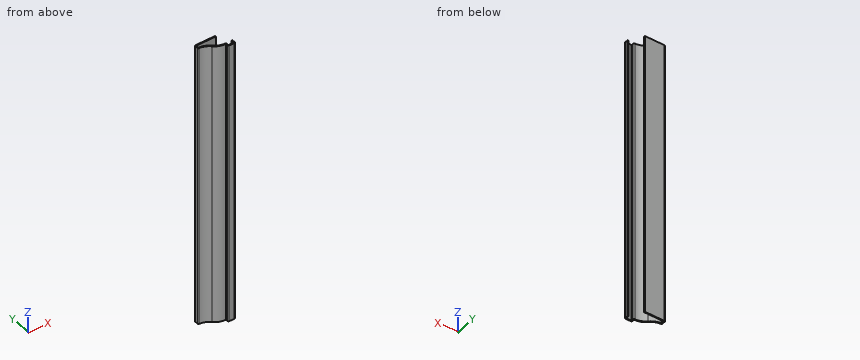
from build123d import *

# Parameters (mm, degrees)
EXTRUDE_THIN1_DEPTH = 285.75
FILLET1_R           = 0.889


with BuildPart() as part:
    # Sketch1 → Extrude-Thin1 (new body)
    with BuildSketch(Plane.XY):
        with BuildLine():
            Line((0, 3.96875), (0, 0))
            Line((0, 0), (-7.14375, 0))
            Line((-7.14375, 0), (-7.14375, 3.175))
            ThreePointArc((-7.14375, 3.175), (-12.992038746, 4.269087389), (-17.962061345, 7.539925789))
            ThreePointArc((-17.962061345, 7.539925789), (-22.83698523, 10.772017174), (-28.575, 11.90625))
            Line((-28.575, 11.90625), (-28.575, 16.66875))
            Line((-28.575, 16.66875), (-7.9375, 16.66875))
            Line((-7.9375, 16.66875), (-7.9375, 15.77975))
            Line((-7.9375, 15.77975), (-27.686, 15.77975))
            Line((-27.686, 15.77975), (-27.686, 12.770487263))
            ThreePointArc((-27.686, 12.770487263), (-22.089870787, 11.419244899), (-17.33645654, 8.171542467))
            ThreePointArc((-17.33645654, 8.171542467), (-12.238465129, 4.931402679), (-6.25475, 4.104858346))
            Line((-6.25475, 4.104858346), (-6.25475, 0.889))
            Line((-6.25475, 0.889), (-0.889, 0.889))
            Line((-0.889, 0.889), (-0.889, 3.96875))
            Line((-0.889, 3.96875), (0, 3.96875))
        make_face()
    extrude(amount=-EXTRUDE_THIN1_DEPTH)

    # Fillet1
    fillet1_edges = [part.edges().sort_by_distance(p)[0] for p in [
        (-6.25475, 4.104858346, -142.875),
        (0, 0, -142.875),
        (-7.14375, 0, -142.875),
        (-28.575, 11.90625, -142.875),
        (-28.575, 16.66875, -142.875),
    ]]
    fillet(fillet1_edges, radius=FILLET1_R)


solid = part.part
Check sheet for the modelled part. Datum: model origin and axes. Units: mm. Give positions to 0.01 mm unless a question says otherwise; leave off trailing zeros. Loops run counter-clockwise (first coordinate to the right, second up) from the corner with the lowest first, then second, coordinate; pieces in that order, holes last. Notation, with made-up numbers: M 89.5,44.25 L 134.5,44.25 A27 cw 134.5,80.25 Z; hole C 85,36.25 d10. An arc over 180 degrees is marked long. Answer as a JSON object with one key per item and string values. Group by question number.
Q1. Material ranges on line 1 along Y through (x, z) = (-8.5, -105.5); line 2 along Y through (x, z) = (-27.25, -38.5); line 3 along Y through (x, z) = (-1.25, -104), recorded low to high. Write a range as [from, to].
Q2. Go/stop test with flat-tipped pins: P1, Ø4, axis at y = 11.5, z = -176.5, coming from the +X side; P2, Ø6, axis at x = -4.5, z = -206, coming from the +Y side; P3, Ø1.5, axis at y = 9, z = -82, coming from the -X side. Record where each tip stops, or that it passes through.
Q3. Cross-section at C-C on x = -22. Record the cut outline in (y, z).
Q4. Cross-section at A-A on x = -10.5. Record the cut outline in (y, z), then the cut area to 3 significant figures.
Q5. Cross-section at B-B on z = -196. Record the cut outline in (x, y) (1 decimal), then the cut area to 3 significant figures.
Evaluation:
{
 "1": {"line 1": "y = [3.22, 4.11], [15.78, 16.67]", "line 2": "y = [11.85, 12.74], [15.78, 16.67]", "line 3": "y = [0, 0.89]"},
 "2": {"P1": "stops at x = -18.86", "P2": "stops at y = 4.06", "P3": "stops at x = -20.8"},
 "3": {"outline": "M 10.4,-285.75 L 11.38,-285.75 L 11.38,0 L 10.4,0 Z; M 15.78,-285.75 L 16.67,-285.75 L 16.67,0 L 15.78,0 Z"},
 "4": {"outline": "M 3.51,-285.75 L 4.42,-285.75 L 4.42,0 L 3.51,0 Z; M 15.78,-285.75 L 16.67,-285.75 L 16.67,0 L 15.78,0 Z", "area": "514 mm2"},
 "5": {"outline": "M -28.6,12.8 A0.9 ccw -27.7,11.9 A15.1 cw -18,7.5 A15.1 ccw -7.1,3.2 L -7.1,0.9 A0.9 ccw -6.3,0 L -0.9,0 A0.9 ccw 0,0.9 L 0,4 L -0.9,4 L -0.9,0.9 L -6.3,0.9 L -6.3,3.2 A0.9 ccw -7.2,4.1 A14.2 cw -17.3,8.2 A16 ccw -27.7,12.8 L -27.7,15.8 L -7.9,15.8 L -7.9,16.7 L -27.7,16.7 A0.9 ccw -28.6,15.8 Z", "area": "53.2 mm2"}
}
